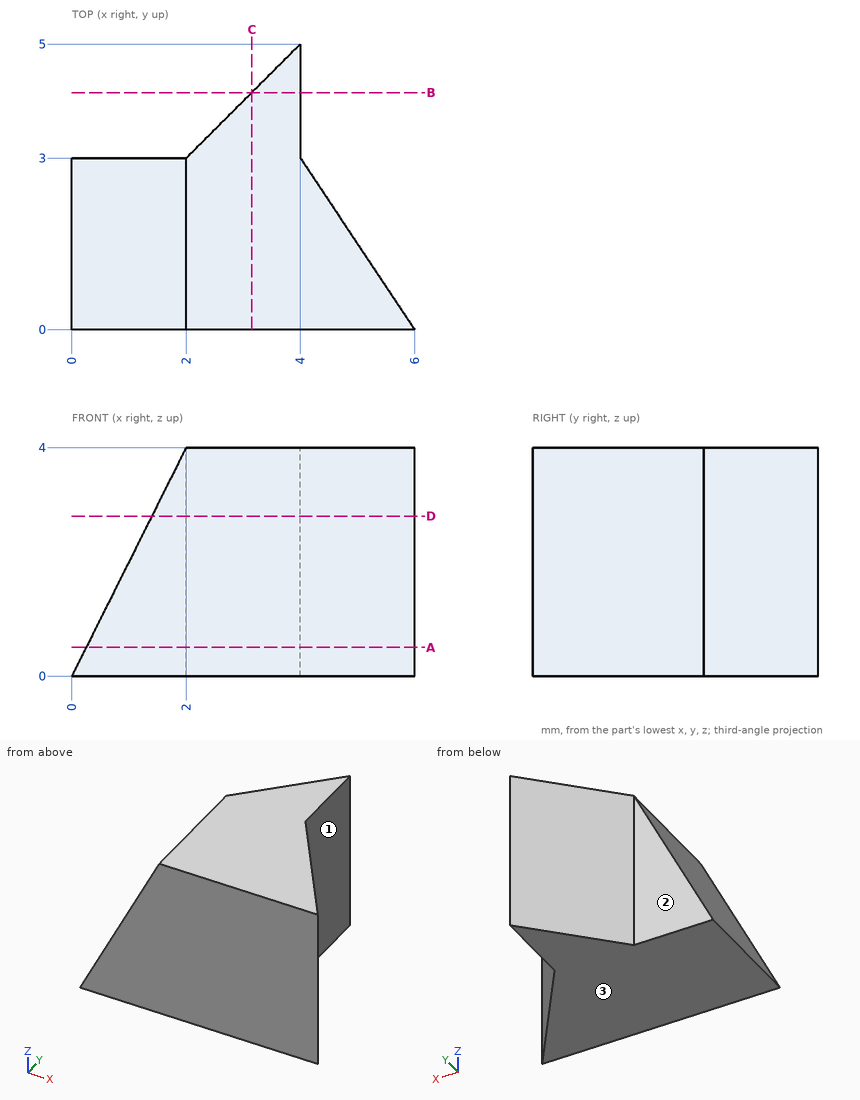
The figure shows three views and two pictorial views of one solid part (mm, origin at its lowest corner). Answer the questions. A direction names the side the tool comes from. Give positions to 0.01 mm unless a question says otherwise; leave off trailing zeros. Order: outer loops, then holes, each group sorted by start corner. A loop starts at its lowest first (then second) coordinate and runs counter-clockwise, first axis right, second up. Notation, with made-up numbers: M 15.25,-9 L 61.25,-9 A28 cw 61.25,17 Z; hole C 8,53 d5. An arc over 180 degrees is marked long. Return JSON: item names as keys, results as strings.
1) Section A-A, the plane z = 0.5 is taken. Write down the section's boundary in (x, y).
Resolved:
{"outline": "M 0.25,0 L 6,0 L 4,3 L 4,5 L 2,3 L 0.25,3 Z"}
2) Section C-C, the plane x = 3.15 is taken. Write down the section's boundary in (y, z).
Resolved:
{"outline": "M 0,0 L 4.15,0 L 4.15,4 L 0,4 Z"}
3) Section D-D, the plane z = 2.8 is taken. Write down the section's boundary in (x, y).
Resolved:
{"outline": "M 1.4,0 L 6,0 L 4,3 L 4,5 L 2,3 L 1.4,3 Z"}
4) A tool of negligible diameter and unlimited length cuts with its end or side. For the marked faces 1, 2 and 3, from which of +Z, -Z, +X, -X, +Y, -Y can it reach the whole face along a straight path? Write none if from no direction.
Resolved:
{"face 1": "+Z, -Z, +X, +Y", "face 2": "+Z, -Z, -X, +Y", "face 3": "-Z, +X, -X, +Y, -Y"}
5) Straight lines are drawn through the part: line 1 along Y through (x, z) = (1.65, 2.05); line 2 along X through (y, z) = (4.1, 2.05); line 3 along X through (y, z) = (2.1, 2.3). For each, find the intervals that lie inside material, in ascending order. Write a range as [from, to].
Resolved:
{"line 1": "[0, 3]", "line 2": "[3.1, 4]", "line 3": "[1.15, 4.6]"}
6) Each of these flat-tipped pins is pushed along its axis until it touches: pin 1 (1.5 mm diameter, centred on x = 2.5, y = 4, fed in from -Z); pin 2 (1.6 mm diameter, centred on x = 1, z = 2.5, fed in from +Y); pin 3 (1.6 mm diameter, centred on y = 4, z = 1.5, fed in from +X); pin 4 (1.5 mm diameter, centred on y = 2, z = 1, fed in from +X). Where does it stop, or does it pass through?
Resolved:
{"pin 1": "z = 0", "pin 2": "y = 3", "pin 3": "x = 4", "pin 4": "x = 5.17"}
7) Section B-B, the plane y = 4.15 is taken. Write down the section's boundary in (x, z).
Resolved:
{"outline": "M 3.15,0 L 4,0 L 4,4 L 3.15,4 Z"}
